from build123d import *

# Parameters (mm, degrees)
ESBO_O1_W                = 55.3
ESBO_O1_H                = 30
RESSALTO_EXTRUS_O1_DEPTH = 1.26
CORTE_EXTRUS_O1_DEPTH    = 63.925969202
CORTE_EXTRUS_O2_DEPTH    = 63.925969202


with BuildPart() as part:
    # Esboço1 → Ressalto-extrusão1 (new body)
    with BuildSketch(Plane(origin=(0, 0, 0), x_dir=(1, 0, 0), z_dir=(0, 1, 0))):
        with Locations((27.65, 15)):
            Rectangle(ESBO_O1_W, ESBO_O1_H)
    extrude(amount=RESSALTO_EXTRUS_O1_DEPTH)

    # Esboço2 → Corte-extrusão1 (cut, through all)
    with BuildSketch(Plane.ZY):
        Polygon((-30, 0), (-29, 1.26), (-30, 1.26), align=None)
    extrude(amount=-CORTE_EXTRUS_O1_DEPTH, mode=Mode.SUBTRACT)

    # Esboço3 → Corte-extrusão2 (cut, through all)
    with BuildSketch(Plane.XY):
        Polygon((0, 1.26), (0, 0), (3.74, 1.26), align=None)
        Polygon((55.3, 1.26), (51.56, 1.26), (55.3, 0), align=None)
    extrude(amount=-CORTE_EXTRUS_O2_DEPTH, mode=Mode.SUBTRACT)


solid = part.part
Verification items for the finished model (mm, model axes). Coordinates: 2 decimals unless noted, no trailing zeros. Order: outer loops, then holes, each group sorted by start corner. A loop starts at its lowest first (then second) coordinate and runs counter-clockwise, first axis right, second up. Notation, with made-up numbers: M 12.25,44 L 25.25,44 A14 ccw 25.25,66 Z; hole C 40.5,-25 d6. An arc over 180 degrees is marked long. One line per item, written item: value. Start each with the question number.
Item 1: Gauge pin test, flat end, axial feed: pin 1 (1 mm diameter, centred on x = 28.5, z = -10.5, fed in from -Y). Record the tip position at first contact, or that the pin passes through.
Item 2: Sectioned sample at A-A (x = 17.5). Enter the section's corners in (y, z).
Item 3: Scan lines: probe 1 along Z at (x, y) = (50, 0.95); probe 2 along Z at (x, y) = (23.5, 0.5). Record each from-to range of solid material in increasing order.
Item 4: Sectioned sample at B-B (z = -8). Enter the section's corners in (x, y), then the cut area to 3 significant figures.
Conclusion:
1. pin 1: stops at y = 0
2. outline: M 0,-30 L 1.26,-29 L 1.26,0 L 0,0 Z
3. probe 1: z = -29.25 to 0
3. probe 2: z = -29.6 to 0
4. outline: M 0,0 L 55.3,0 L 51.56,1.26 L 3.74,1.26 Z
4. area: 65.0 mm^2
